from build123d import *

# Parameters (mm, degrees)
SKETCH625_W             = 1120
SKETCH625_H             = 650
PAD299_DEPTH            = 50
SKETCH626_W             = 1070
SKETCH626_H             = 600
POCKET007_DEPTH         = 20
FILLET210_R             = 5
BODY126_PLACEMENT_ANGLE = 90


with BuildPart() as part:
    # Sketch625 → Pad299 (new body)
    with BuildSketch(Plane.XZ):
        with Locations((560, 325)):
            Rectangle(SKETCH625_W, SKETCH625_H)
    extrude(amount=PAD299_DEPTH)

    # Sketch626 (on Face6 of Pad299) → Pocket007 (cut)
    with BuildSketch(Plane.XZ.offset(50)):
        with Locations((560, 325)):
            Rectangle(SKETCH626_W, SKETCH626_H)
    extrude(amount=-POCKET007_DEPTH, mode=Mode.SUBTRACT)

    # Fillet210
    fillet210_edges = [part.edges().sort_by_distance(p)[0] for p in [
        (560, -50, 0),
        (0, -50, 325),
        (1120, -50, 325),
        (560, -50, 650),
        (25, -50, 325),
        (560, -50, 25),
        (1095, -50, 325),
        (560, -50, 625),
    ]]
    fillet(fillet210_edges, radius=FILLET210_R)


with BuildPart() as part_1:
    # Body126 placement: moved
    add(part.part.moved(Location((1641, 1679, 1299))).rotate(Axis((1641, 1679, 1299), (0, 0, 1)), BODY126_PLACEMENT_ANGLE))


solid = part_1.part
Here's how the part is built. I have some questions about the finished solid (model axes, mm). Round coordinates to 2 decimals unless told otherwise and drop trailing zeros. Loops run counter-clockwise (first coordinate to the right, second up) from the corner with the lowest first, then second, coordinate; pieces in that order, holes last. Notation, with made-up numbers: (13, 19) - (50, 19) arc R10 cw to (50, 32) - close; hole circle Ø10 at (-39.5, 31). An arc over 180 degrees is marked (long way). One line per question, with ' | ' between items. Start each with the question number.
Q1. I want a section at A-A (y = 2039). Write out the boundary of the cut face in (x, z).
Q2. We'd pull the mould along Y, two halves only. Please class faces 1 (the flat face through (1691, 2236, 1317)), 2 (the flat face through (1671, 2232, 1628)), 3 (the flat face through (1663, 2799, 1619)): +Y half, -Y half, draft (parallel to the pull), parting line (faces both ways), or undercut.
Q3. Please list where these lines run through material, in increasing order: line 1 (Z direction, x = 1673.5, y = 2318); line 2 (Y direction, x = 1680.5, z = 1395); line 3 (X direction, y = 1814, z = 1544). Write a range as [from, to].
Q4. I want a section at B-B (z = 1894). Write out the boundary of the cut face in (x, y).
Q5. Will this pin go through, and if not, where does the flat tip stop? pin 1 (6 mm diameter, centred on y = 2643.5, z = 1809, fed in from +X).
Response values:
1) outline: (1641, 1299) - (1686, 1299) arc R5 ccw to (1691, 1304) - (1691, 1319) arc R5 ccw to (1686, 1324) - (1671, 1324) - (1671, 1924) - (1686, 1924) arc R5 ccw to (1691, 1929) - (1691, 1944) arc R5 ccw to (1686, 1949) - (1641, 1949) - close
2) face 1: draft | face 2: undercut | face 3: +Y half
3) line 1: z = [1299, 1324], [1924, 1949] | line 2: y = [1679, 1704], [2774, 2799] | line 3: x = [1641, 1671]
4) outline: (1641, 1679) - (1686, 1679) arc R5 ccw to (1691, 1684) - (1691, 1699) arc R5 ccw to (1686, 1704) - (1671, 1704) - (1671, 2774) - (1686, 2774) arc R5 ccw to (1691, 2779) - (1691, 2794) arc R5 ccw to (1686, 2799) - (1641, 2799) - close
5) pin 1: stops at x = 1671
